Source: three-view drawing plus pictorial views. Frame: mm from the lowest corner of the part. A direction names the side the tool comes from. Round coordinates to 2 decimals unless told otherwise and drop trailing zeros. Write each loop counter-clockwise with the first axis right and the second up, starting at its lowest first coordinate (ties: lowest second). Pieces come first, ordered by that corner, then holes. Notation, with made-up numbers: (13.5, -40) -> (71.5, -40) arc R12 ccw to (71.5, -34) -> close; hole circle Ø9 at (3.25, 49.5). An arc over 180 degrees is marked (long way). Put each result on its own line as item: value.
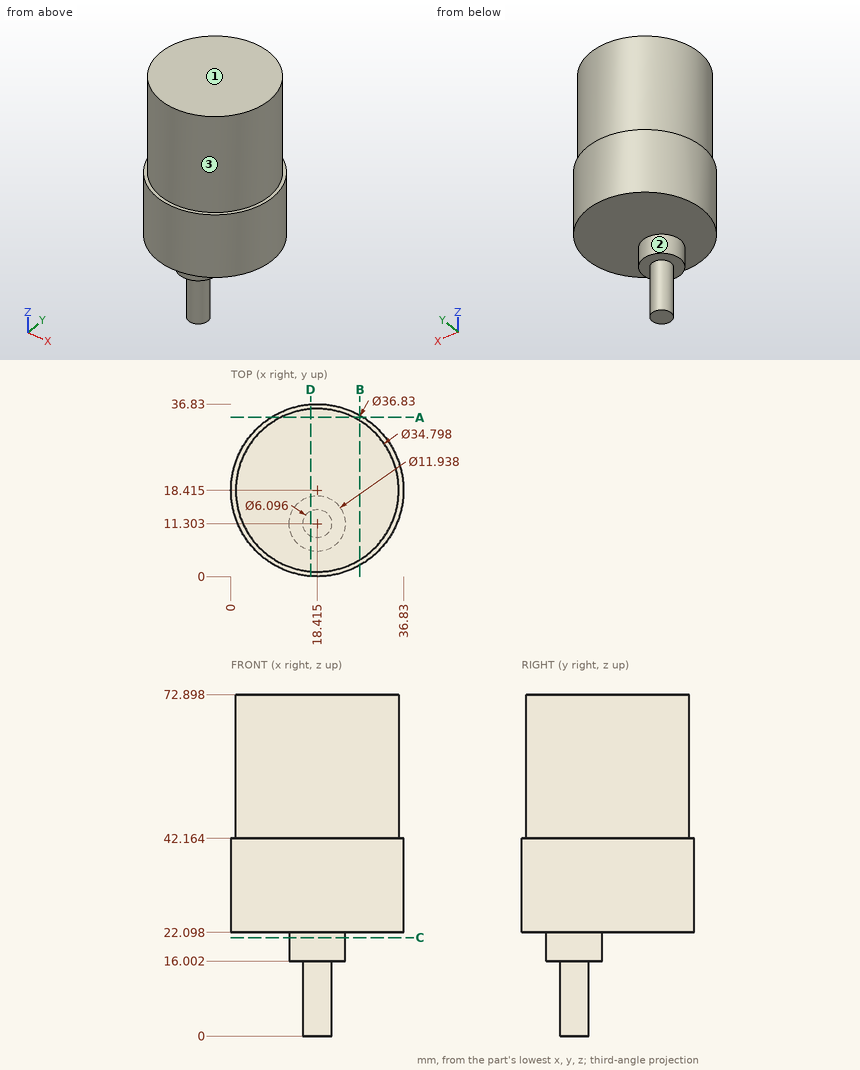
Q1. Cut plane C-C on z = 21. Output: boundary loops of the cut face in (x, y) (3 decimals).
Ans:
outline: circle Ø11.938 at (18.415, 11.303)
Q2. Reachability of the marked faces 1, 2 and 3 from +Z, -Z, +X, -X, +Y, -Y: full face, straight path, thin tool, end or side. Return the list, or none.
Ans:
face 1: +Z, +X, -X, +Y, -Y
face 2: -Z
face 3: +Z
Q3. Cut plane D-D on x = 17. Output: boundary loops of the cut face in (y, z), and give its area (3 significant figures).
Ans:
outline: (0.05, 22.1) -> (5.5, 22.1) -> (5.5, 16) -> (8.6, 16) -> (8.6, 0) -> (14, 0) -> (14, 16) -> (17.1, 16) -> (17.1, 22.1) -> (36.78, 22.1) -> (36.78, 42.16) -> (35.76, 42.16) -> (35.76, 72.9) -> (1.07, 72.9) -> (1.07, 42.16) -> (0.05, 42.16) -> close
area: 1,960 mm^2
Q4. Pin query (flat end, axial travel): pin 1 (10 mm diameter, centred on y = 11.5, z = 30, fed in from +X); pin 2 (5 mm diameter, centred on x = 17, z = 38.5, fed in from -Y); pin 3 (10 mm diameter, centred on x = 7, y = 30, fed in from -Z). Return the tip coordinate at first contact, or that it passes through.
Ans:
pin 1: stops at x = 36.73
pin 2: stops at y = 0
pin 3: stops at z = 22.1
Q5. Cut plane A-A on y = 34. Output: boundary loops of the cut face in (x, z), and give its area (3 significant figures).
Ans:
outline: (8.61, 22.1) -> (28.22, 22.1) -> (28.22, 42.16) -> (26.15, 42.16) -> (26.15, 72.9) -> (10.68, 72.9) -> (10.68, 42.16) -> (8.61, 42.16) -> close
area: 869 mm^2
Q6. Cut plane B-B on x = 27.5. Output: boundary loops of the cut face in (y, z).
Ans:
outline: (2.4, 22.1) -> (34.43, 22.1) -> (34.43, 42.16) -> (33.25, 42.16) -> (33.25, 72.9) -> (3.58, 72.9) -> (3.58, 42.16) -> (2.4, 42.16) -> close
Q7. Material intervals for line 1 (Z direction, x = 8, y = 11); line 2 (X direction, y = 19, z = 25.5); line 3 (Z direction, x = 20, y = 8), sorted ascending. Write a range as [from, to].
Ans:
line 1: z = [22.1, 72.9]
line 2: x = [0.01, 36.82]
line 3: z = [16, 72.9]
